The model under review builds one solid part; all positions refer to its coordinate system, in mm. Coordinates: 2 decimals unless noted, no trailing zeros. Loops run counter-clockwise (first coordinate to the right, second up) from the corner with the lowest first, then second, coordinate; pieces in that order, holes last. Notation, with made-up numbers: (9.5, 18) - (13.5, 18) arc R22 ccw to (13.5, 42) - close; hole circle Ø3 at (24, -16). An arc over 180 degrees is marked (long way). Answer in a Markdown table with one row per item. Add a question column.
(1) For line 1 along Y through (x, z) = (0, 6.5); line 2 along X through (y, z) = (-12.5, 10); line 3 along X through (y, z) = (-2.5, 5), list the stretches that pass through material, from the lowest coordinate up.
(2) Mouldability with a two-part tool opening along X and no side actions: class faces 1 (the conical face through (-0.317, -22.384, 0.187)), 2 (the cylindrical face through (-4.336, -19.524, 7.888)), 3 (the flat face through (-7, 19, 0)) as +X half, -X half, draft (parallel to the pull), parting line (faces both ways), or undercut.
(3) We need section C-C on z = 8.75. Write out the cut boundary in (x, y), plus the area to 3 significant figures.
(4) We need section A-A on x = 0. Write out the cut boundary in (y, z), plus the area to 3 significant figures.
(5) We need section B-B on y = 0. Write out the cut boundary in (x, z), plus the area to 3 significant figures.
(6) For P1, Ø4, axis at x = -0.5, z = 6.5, coming from the -Y side; P2, Ø0.8, axis at y = 23, z = 10, coming from the +X side; P3, Ø1, axis at y = -11.5, z = 5, coming from the +X side, all flat-tipped, find the tip position at first contact; note any pin that passes through.
from build123d import *

# Parameters (mm, degrees)
SKETCH1_R      = 22.5
SKETCH1_R_2    = 20
EXTRUDE1_DEPTH = 16
EXTRUDE2_DEPTH = 16
CHAMFER1_SIZE  = 0.5
CHAMFER1_SIZE2 = 0.181985117
FILLET1_R      = 0.4


with BuildPart() as part:
    # Sketch1 → Extrude1 (new body)
    with BuildSketch(Plane.XY):
        Circle(SKETCH1_R)
        Circle(SKETCH1_R_2, mode=Mode.SUBTRACT)
    extrude(amount=EXTRUDE1_DEPTH)

    # Sketch3 → Extrude2 (add)
    with BuildSketch(Plane.XY.offset(16)):
        with BuildLine():
            Line((2.5, 25), (2.5, 22.360679775))
            ThreePointArc((2.5, 22.360679775), (0, 22.5), (-2.5, 22.360679775))
            Line((-2.5, 22.360679775), (-2.5, 25))
            ThreePointArc((-2.5, 25), (0, 27.5), (2.5, 25))
        make_face()
    extrude(amount=-EXTRUDE2_DEPTH)

    # Chamfer1
    chamfer1_edges = [part.edges().sort_by_distance(p)[0] for p in [
        (0, -22.5, 0),
    ]]
    chamfer1_side = [part.faces().sort_by_distance(p)[0] for p in [
        (0, -22.5, 8),
    ]]
    chamfer(chamfer1_edges, length=CHAMFER1_SIZE, length2=CHAMFER1_SIZE2, reference=chamfer1_side[0])

    # Fillet1
    fillet1_edges = [part.edges().sort_by_distance(p)[0] for p in [
        (2.5, 22.360679775, 8.25),
        (-2.5, 22.360679775, 8.25),
    ]]
    fillet(fillet1_edges, radius=FILLET1_R)


solid = part.part
Outcome:
| question | item | result |
|---|---|---|
| 1 | line 1 | -22.5 to -20, 20 to 27.5 |
| 1 | line 2 | -18.71 to -15.61, 15.61 to 18.71 |
| 1 | line 3 | -22.36 to -19.84, 19.84 to 22.36 |
| 2 | face 1 | parting line |
| 2 | face 2 | undercut |
| 2 | face 3 | draft |
| 3 | outline | (-2.85, 22.32) arc R22.5 ccw (long way) to (2.85, 22.32) arc R0.4 cw to (2.5, 22.72) - (2.5, 25) arc R2.5 ccw to (-2.5, 25) - (-2.5, 22.72) arc R0.4 cw to start; hole circle Ø40 at (0, 0) |
| 3 | area | 356 mm² |
| 4 | outline | (-22.5, 0.5) - (-22.32, 0) - (-20, 0) - (-20, 16) - (-22.5, 16) - close; (20, 0) - (27.5, 0) - (27.5, 16) - (20, 16) - close |
| 4 | area | 160 mm² |
| 5 | outline | (-22.5, 0.5) - (-22.32, 0) - (-20, 0) - (-20, 16) - (-22.5, 16) - close; (20, 0) - (22.32, 0) - (22.5, 0.5) - (22.5, 16) - (20, 16) - close |
| 5 | area | 79.9 mm² |
| 6 | P1 | y = -22.5 |
| 6 | P2 | x = 2.52 |
| 6 | P3 | x = 19.63 |
